Geometry: see drawing. Coordinates: mm, zero at the bounding-box minimum. A direction names the side the tool comes from. Coordinates: 2 decimals unless noted, no trailing zeros. Write each loop counter-clockwise with the first axis right and the second up, starting at its lowest first coordinate (ties: lowest second). Pieces come first, ordered by that corner, then holes.
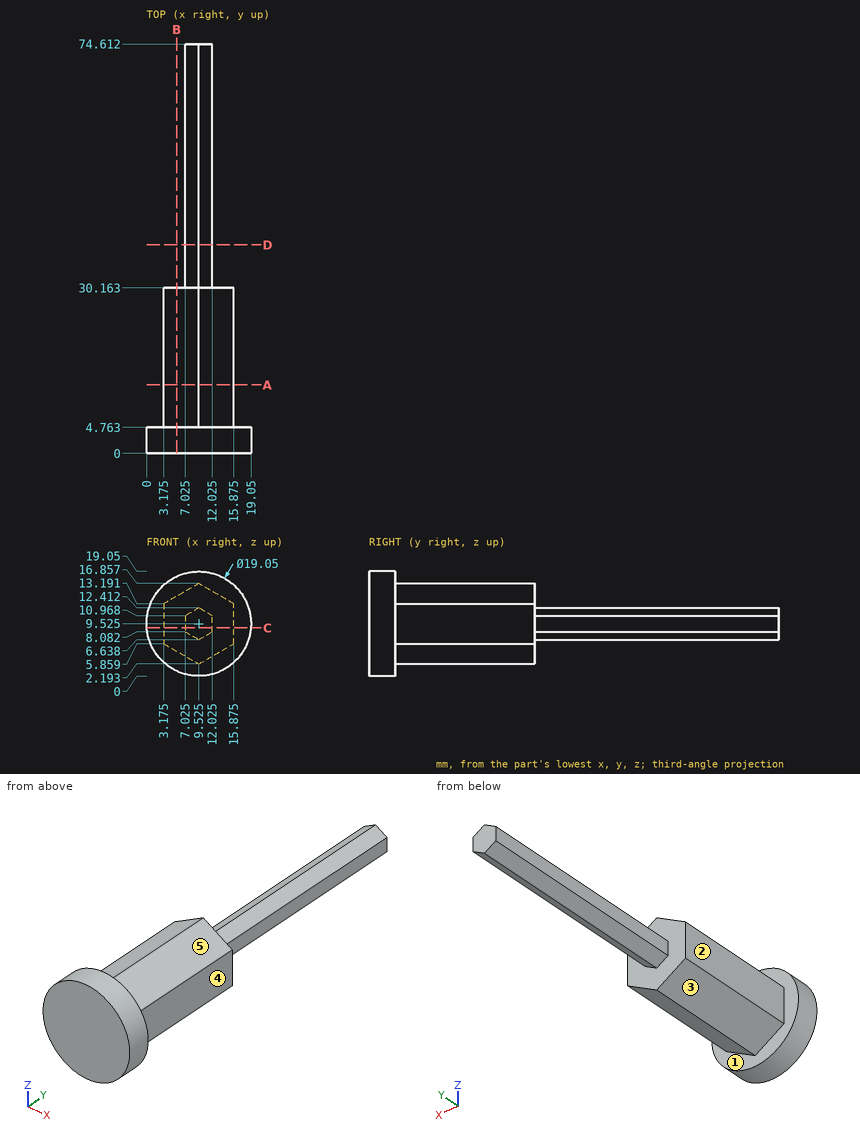
Item 1: Set-up query: the marked faces 1, 2, 3, 4 and 5. Return all of +Z, -Z, +X, -X, +Y, -Y with unobstructed straight access to the full face (end or side cutting, diameter ignored); none if empty.
Derived:
face 1: +Y
face 2: +Z, -Z, -X, +Y
face 3: -Z, -X, +Y
face 4: +Z, -Z, +X, +Y
face 5: +Z, +X, +Y
Item 2: Section A-A, the plane y = 12.5. Output: boundary loops of the cut face in (x, z) (1 decimal).
Derived:
outline: (3.2, 5.9) - (9.5, 2.2) - (15.9, 5.9) - (15.9, 13.2) - (9.5, 16.9) - (3.2, 13.2) - close
Item 3: Section B-B, the plane x = 5.5. Output: boundary loops of the cut face in (y, z), plus the area to 3 significant figures.
Derived:
outline: (0, 0.89) - (4.76, 0.89) - (4.76, 4.52) - (30.16, 4.52) - (30.16, 14.53) - (4.76, 14.53) - (4.76, 18.16) - (0, 18.16) - close
area: 337 mm2
Item 4: Pin query (flat end, axial travel): pin 1 (1 mm diameter, centred on y = 7.5, z = 11, fed in from +X) (1 decimal); pin 2 (0.9 mm diameter, centred on y = 41.5, z = 9, fed in from -X) (1 decimal); pin 3 (2 mm diameter, centred on x = 3.5, y = 12, fed in from -Z) (1 decimal). Return the tip coordinate at first contact, or that it passes through.
Derived:
pin 1: stops at x = 15.9
pin 2: stops at x = 7
pin 3: stops at z = 5.1
Item 5: Material intervals for probe 1 along X at (y, z) = (29, 8.5) (1 decimal); probe 2 along Y at (x, z) = (1, 12.75); probe 3 along Y at (x, z) = (7.5, 6.75), sorted ascending.
Derived:
probe 1: x = 3.2 to 15.9
probe 2: y = 0 to 4.76
probe 3: y = 0 to 30.16
Item 6: Section C-C, the plane z = 8.75. Output: boundary loops of the cut face in (x, y) (1 decimal), plus the area to 3 significant figures.
Derived:
outline: (0, 0) - (19, 0) - (19, 4.8) - (15.9, 4.8) - (15.9, 30.2) - (12, 30.2) - (12, 74.6) - (7, 74.6) - (7, 30.2) - (3.2, 30.2) - (3.2, 4.8) - (0, 4.8) - close
area: 635 mm2
Item 7: Section D-D, the plane y = 38. Output: boundary loops of the cut face in (x, z) (1 decimal).
Derived:
outline: (7, 8.1) - (9.5, 6.6) - (12, 8.1) - (12, 11) - (9.5, 12.4) - (7, 11) - close
